Design review of the part built by this model. Coordinates are the model's own, in mm. Face numbers are marked on the shaded views. A direction names the side the tool comes from. Coordinates: 2 decimals unless noted, no trailing zeros. Write each loop counter-clockwise with the first axis right and the second up, starting at its lowest first coordinate (ties: lowest second). Pieces come first, ordered by that corner, then holes.
Q1. Machinability: for the marked faces 1, 2 and 3, which of the approach directions +Z, -Z, +X, -X, +Y, -Y give a long, thin tool a straight path to every point of the face, cutting with its end or side? Answer none if there is none.
Q2. Mouldability with a two-part tool opening along X and no side actions: class the marked faces 4 and 5 as pulls with the +X half, pulls with the -X half, needs draft (parallel to the pull), parting line crosses it, or undercut.
Q3. For probe 1 along Y at (x, z) = (0, 289); probe 2 along X at (y, z) = (-5.5, 291); probe 3 along X at (y, z) = (-5.75, 293), list the stretches that pass through material, from the lowest coordinate up.
Q4. Insertion check: pin 1 (1.8 mm diameter, centred on x = -5.5, z = 286, fed in from -Y); pin 2 (6 mm diameter, centred on x = 0, z = 300, fed in from -Y); pin 3 (3.5 mm diameter, centred on y = -0.5, z = 286, fed in from +X); pin 4 (1.7 mm diameter, centred on x = 0, z = 295, fed in from -Y). Each pin has a flat end and moves straight along its axis. Give the tip position at first contact, or say it passes through.
Q5. Take a section at A-A (y = 0). Give the boundary of the cut face in (x, z), and give its area (3 significant figures).
Q6. Take a section at B-B (x = 0). Give the boundary of the cut face in (y, z), and give its area (3 significant figures).
```python
from build123d import *

# Parameters (mm, degrees)
SKETCH1_R           = 2.6035
BOSS_EXTRUDE1_DEPTH = 304.8
SKETCH2_R           = 24.282664684
CUT_EXTRUDE1_DEPTH  = 577.85


with BuildPart() as part:
    # Sketch1 → Boss-Extrude1 (new, symmetric)
    with BuildSketch(Plane.XY):
        with BuildLine():
            Line((-7.179650497, -8.645192506), (-3.952270251, -5.423690499))
            ThreePointArc((-3.952270251, -5.423690499), (-2.922936451, -4.736929036), (-1.709253557, -4.4958))
            Line((-1.709253557, -4.4958), (1.709253557, -4.4958))
            ThreePointArc((1.709253557, -4.4958), (2.922936451, -4.736929036), (3.952270251, -5.423690499))
            Line((3.952270251, -5.423690499), (7.179650497, -8.645192506))
            ThreePointArc((7.179650497, -8.645192506), (7.41473083, -9.822813117), (6.416408329, -10.4902))
            Line((6.416408329, -10.4902), (4.287512407, -10.4902))
            ThreePointArc((4.287512407, -10.4902), (3.54574862, -10.79744862), (3.2385, -11.539212407))
            Line((3.2385, -11.539212407), (3.2385, -11.650987593))
            ThreePointArc((3.2385, -11.650987593), (3.54574862, -12.39275138), (4.287512407, -12.7))
            Line((4.287512407, -12.7), (5.317126718, -12.7))
            ThreePointArc((5.317126718, -12.7), (5.825126718, -12.192), (6.333126718, -12.7))
            Line((6.333126718, -12.7), (9.550443118, -12.7))
            ThreePointArc((9.550443118, -12.7), (10.058366869, -12.192000006), (10.566443095, -12.699847501))
            ThreePointArc((10.566443095, -12.699847501), (12.082537762, -12.08250727), (12.699846982, -10.566399977))
            ThreePointArc((12.699846982, -10.566399977), (12.192000006, -10.058323491), (12.7, -9.5504))
            Line((12.7, -9.5504), (12.7, -6.3330836))
            ThreePointArc((12.7, -6.3330836), (12.192, -5.8250836), (12.7, -5.3170836))
            Line((12.7, -5.3170836), (12.7, -4.287469289))
            ThreePointArc((12.7, -4.287469289), (12.39275138, -3.545705502), (11.650987593, -3.238456882))
            Line((11.650987593, -3.238456882), (11.539212407, -3.238456882))
            ThreePointArc((11.539212407, -3.238456882), (10.79744862, -3.545705502), (10.4902, -4.287469289))
            Line((10.4902, -4.287469289), (10.4902, -6.402089023))
            ThreePointArc((10.4902, -6.402089023), (9.856505071, -7.351067942), (8.737131347, -7.129408934))
            Line((8.737131347, -7.129408934), (5.441005833, -3.840816462))
            ThreePointArc((5.441005833, -3.840816462), (4.750877967, -2.809883091), (4.5085, -1.593185507))
            Line((4.5085, -1.593185507), (4.5085, 1.593185507))
            ThreePointArc((4.5085, 1.593185507), (4.750877967, 2.809883091), (5.441005833, 3.840816462))
            Line((5.441005833, 3.840816462), (8.737131347, 7.129408934))
            ThreePointArc((8.737131347, 7.129408934), (9.856505071, 7.351067942), (10.4902, 6.402089023))
            Line((10.4902, 6.402089023), (10.4902, 4.287469289))
            ThreePointArc((10.4902, 4.287469289), (10.79744862, 3.545705502), (11.539212407, 3.238456882))
            Line((11.539212407, 3.238456882), (11.650987593, 3.238456882))
            ThreePointArc((11.650987593, 3.238456882), (12.39275138, 3.545705502), (12.7, 4.287469289))
            Line((12.7, 4.287469289), (12.7, 5.3170836))
            ThreePointArc((12.7, 5.3170836), (12.192, 5.8250836), (12.7, 6.3330836))
            Line((12.7, 6.3330836), (12.7, 9.5504))
            ThreePointArc((12.7, 9.5504), (12.192000006, 10.058323491), (12.699846982, 10.566399977))
            ThreePointArc((12.699846982, 10.566399977), (12.082537762, 12.08250727), (10.566443095, 12.699847501))
            ThreePointArc((10.566443095, 12.699847501), (10.058366869, 12.192000006), (9.550443118, 12.7))
            Line((9.550443118, 12.7), (6.333126718, 12.7))
            ThreePointArc((6.333126718, 12.7), (5.825126718, 12.192), (5.317126718, 12.7))
            Line((5.317126718, 12.7), (4.287512407, 12.7))
            ThreePointArc((4.287512407, 12.7), (3.54574862, 12.39275138), (3.2385, 11.650987593))
            Line((3.2385, 11.650987593), (3.2385, 11.539212407))
            ThreePointArc((3.2385, 11.539212407), (3.54574862, 10.79744862), (4.287512407, 10.4902))
            Line((4.287512407, 10.4902), (6.476788598, 10.4902))
            ThreePointArc((6.476788598, 10.4902), (7.432222385, 9.85140422), (7.207036008, 8.724370562))
            Line((7.207036008, 8.724370562), (3.898272566, 5.423169045))
            ThreePointArc((3.898272566, 5.423169045), (2.869120213, 4.736787962), (1.655778399, 4.4958))
            Line((1.655778399, 4.4958), (-1.655778399, 4.4958))
            ThreePointArc((-1.655778399, 4.4958), (-2.869120213, 4.736787962), (-3.898272566, 5.423169045))
            Line((-3.898272566, 5.423169045), (-7.207036008, 8.724370562))
            ThreePointArc((-7.207036008, 8.724370562), (-7.432222385, 9.85140422), (-6.476788598, 10.4902))
            Line((-6.476788598, 10.4902), (-4.287512407, 10.4902))
            ThreePointArc((-4.287512407, 10.4902), (-3.54574862, 10.79744862), (-3.2385, 11.539212407))
            Line((-3.2385, 11.539212407), (-3.2385, 11.650987593))
            ThreePointArc((-3.2385, 11.650987593), (-3.54574862, 12.39275138), (-4.287512407, 12.7))
            Line((-4.287512407, 12.7), (-5.317126718, 12.7))
            ThreePointArc((-5.317126718, 12.7), (-5.825126718, 12.192), (-6.333126718, 12.7))
            Line((-6.333126718, 12.7), (-9.550443118, 12.7))
            ThreePointArc((-9.550443118, 12.7), (-10.058366869, 12.192000006), (-10.566443095, 12.699847501))
            ThreePointArc((-10.566443095, 12.699847501), (-12.082537762, 12.08250727), (-12.699846982, 10.566399977))
            ThreePointArc((-12.699846982, 10.566399977), (-12.192000006, 10.058323491), (-12.7, 9.5504))
            Line((-12.7, 9.5504), (-12.7, 6.3330836))
            ThreePointArc((-12.7, 6.3330836), (-12.192, 5.8250836), (-12.7, 5.3170836))
            Line((-12.7, 5.3170836), (-12.7, 4.287469289))
            ThreePointArc((-12.7, 4.287469289), (-12.39275138, 3.545705502), (-11.650987593, 3.238456882))
            Line((-11.650987593, 3.238456882), (-11.539212407, 3.238456882))
            ThreePointArc((-11.539212407, 3.238456882), (-10.79744862, 3.545705502), (-10.4902, 4.287469289))
            Line((-10.4902, 4.287469289), (-10.4902, 6.402089023))
            ThreePointArc((-10.4902, 6.402089023), (-9.856505071, 7.351067942), (-8.737131347, 7.129408934))
            Line((-8.737131347, 7.129408934), (-5.441005833, 3.840816462))
            ThreePointArc((-5.441005833, 3.840816462), (-4.750877967, 2.809883091), (-4.5085, 1.593185507))
            Line((-4.5085, 1.593185507), (-4.5085, -1.593185507))
            ThreePointArc((-4.5085, -1.593185507), (-4.750877967, -2.809883091), (-5.441005833, -3.840816462))
            Line((-5.441005833, -3.840816462), (-8.737131347, -7.129408934))
            ThreePointArc((-8.737131347, -7.129408934), (-9.856505071, -7.351067942), (-10.4902, -6.402089023))
            Line((-10.4902, -6.402089023), (-10.4902, -4.287469289))
            ThreePointArc((-10.4902, -4.287469289), (-10.79744862, -3.545705502), (-11.539212407, -3.238456882))
            Line((-11.539212407, -3.238456882), (-11.650987593, -3.238456882))
            ThreePointArc((-11.650987593, -3.238456882), (-12.39275138, -3.545705502), (-12.7, -4.287469289))
            Line((-12.7, -4.287469289), (-12.7, -5.3170836))
            ThreePointArc((-12.7, -5.3170836), (-12.192, -5.8250836), (-12.7, -6.3330836))
            Line((-12.7, -6.3330836), (-12.7, -9.5504))
            ThreePointArc((-12.7, -9.5504), (-12.192000006, -10.058323491), (-12.699846982, -10.566399977))
            ThreePointArc((-12.699846982, -10.566399977), (-12.082537762, -12.08250727), (-10.566443095, -12.699847501))
            ThreePointArc((-10.566443095, -12.699847501), (-10.058366869, -12.192000006), (-9.550443118, -12.7))
            Line((-9.550443118, -12.7), (-6.333126718, -12.7))
            ThreePointArc((-6.333126718, -12.7), (-5.825126718, -12.192), (-5.317126718, -12.7))
            Line((-5.317126718, -12.7), (-4.287512407, -12.7))
            ThreePointArc((-4.287512407, -12.7), (-3.54574862, -12.39275138), (-3.2385, -11.650987593))
            Line((-3.2385, -11.650987593), (-3.2385, -11.539212407))
            ThreePointArc((-3.2385, -11.539212407), (-3.54574862, -10.79744862), (-4.287512407, -10.4902))
            Line((-4.287512407, -10.4902), (-6.416408329, -10.4902))
            ThreePointArc((-6.416408329, -10.4902), (-7.41473083, -9.822813117), (-7.179650497, -8.645192506))
        make_face()
        with Locations(Location((0, 0, 0), (0, 0, 180))):
            Circle(SKETCH1_R, mode=Mode.SUBTRACT)
    extrude(amount=BOSS_EXTRUDE1_DEPTH, both=True)

    # Sketch2 → Cut-Extrude1 (cut)
    with BuildSketch(Plane(origin=(0, 0, -304.8), x_dir=(-1, 0, 0), z_dir=(0, 0, -1))):
        Circle(SKETCH2_R)
    extrude(amount=-CUT_EXTRUDE1_DEPTH, mode=Mode.SUBTRACT)


solid = part.part
```
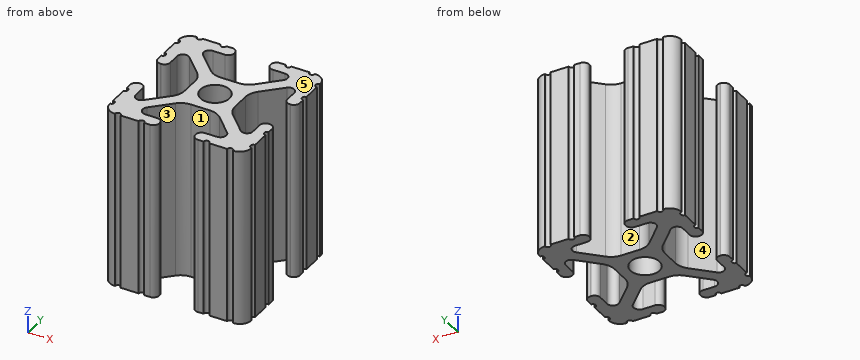
Response:
1. face 1: +Z, -Z, -Y
1. face 2: +Z, -Z, +Y
1. face 3: +Z, -Z
2. face 4: undercut
2. face 5: needs draft
3. probe 1: y = -4.5 to -2.6, 2.6 to 4.5
3. probe 2: x = -12.31 to -10.49, -7.1 to -4.03, 4.03 to 7.1, 10.49 to 12.31
3. probe 3: x = -12.2 to -10.49, -7.35 to -4.28, 4.28 to 7.35, 10.49 to 12.2
4. pin 1: stops at y = -12.7
4. pin 2: stops at y = -4.77
4. pin 3: stops at x = 4.58
4. pin 4: stops at y = -4.5
5. outline: (-4.51, 273.05) - (-2.6, 273.05) - (-2.6, 304.8) - (-4.51, 304.8) - close; (2.6, 273.05) - (4.51, 273.05) - (4.51, 304.8) - (2.6, 304.8) - close
5. area: 121 mm2
6. outline: (-4.5, 273.05) - (-2.6, 273.05) - (-2.6, 304.8) - (-4.5, 304.8) - close; (2.6, 273.05) - (4.5, 273.05) - (4.5, 304.8) - (2.6, 304.8) - close
6. area: 120 mm2
